Check sheet for the modelled part. Datum: model origin and axes. Units: mm. A direction names the side the tool comes from. Give positions to 0.01 mm unless a question says otherwise; leave off trailing zeros. Order: outer loops, then holes, each group sorted by start corner. A loop starts at its lowest first (then second) coordinate and runs counter-clockwise, first axis right, second up.
Item 1: Gauge pin test, flat ends, axial feed: P1, Ø0.6, axis at y = -0.5, z = 16.5, coming from the +X side; P2, Ø1.5, axis at y = 3, z = 7, coming from the +X side; P3, Ø1.6, axis at y = 0.5, z = 16.5, coming from the -X side. Record the tip position at first contact, or that the pin passes through.
Item 2: Sectioned sample at D-D on z = 9.25. Record the boundary of the cut face in (x, y), and give its area (3 significant figures).
Item 3: Material ranges on line 1 along Z through (x, y) = (3.5, 4.75); line 2 along X through (y, z) = (-0.5, 16.5); line 3 along Z through (x, y) = (-1.25, 1), recorded low to high.
Item 4: Sectioned sample at B-B on y = 0. Record the boundary of the cut face in (x, z), and give its area (3 significant figures).
Item 5: Release check for a two-part mould opening along X. For faces 6 (the cylindrical face through (-6, 0, 7)), 7 (the cylindrical face through (6, 0, 7)), 8 (the cylindrical face through (-0.54, -2.44, 15.49)) record: released by +X, released by -X, zero draft, split by the parting line, or undercut.
Item 6: Access from +Z, -Z, +X, -X, +Y, -Y to the whole of each face (thin tool, end or side, straight path). Record for faces 1 (the flat face through (-0.1, -2.2, 0)), 2 (the flat face through (-4.5, 0, 16)), 3 (the flat face through (3, 0, 15)), 4 (the flat face through (4.5, 0, 16)), 5 (the flat face through (4, 0, 16)).
Item 7: Sectioned sample at C-C on x = 0. Record the boundary of the cut face in (y, z), and give its area (3 significant figures).
Item 8: Sectioned sample at A-A on z = 15.5. Record the boundary of the cut face in (x, y), and give its area (3 significant figures).
from build123d import *

# Parameters (mm, degrees)
SKETCH_1_R          = 6
EXTRUDE_1_DEPTH     = 15
CUT_EXTRUDE_1_DEPTH = 15
SKETCH_7_R          = 2.5
EXTRUDE_2_DEPTH     = 1.2
FILLET_1_R          = 0.2
SKETCH_8_R          = 0.5
EXTRUDE_3_DEPTH     = 0.3
FILLET_2_R          = 0.05
EXTRUDE_4_DEPTH     = 2.4
CHAMFER_1_SIZE      = 0.5
CHAMFER_2_SIZE      = 0.5
CHAMFER_3_SIZE      = 0.5
SKETCH_10_R         = 2
EXTRUDE_5_DEPTH     = 0.1


with BuildPart() as part:
    # 草图1 → 凸台-拉伸1 (new body)
    with BuildSketch(Plane.XY):
        Circle(SKETCH_1_R)
    extrude(amount=EXTRUDE_1_DEPTH)

    # 草图6 → 切除-拉伸1 (cut)
    with BuildSketch(Plane(origin=(0, 0, 0), x_dir=(-1, 0, 0), z_dir=(0, 0, -1))):
        with BuildLine():
            Line((-3.31662479, 5), (3.31662479, 5))
            ThreePointArc((3.31662479, 5), (0, 6), (-3.31662479, 5))
        make_face()
        with BuildLine():
            Line((-3.31662479, -5), (3.31662479, -5))
            ThreePointArc((3.31662479, -5), (0, -6), (-3.31662479, -5))
        make_face()
    extrude(amount=-CUT_EXTRUDE_1_DEPTH, mode=Mode.SUBTRACT)

    # 草图7 → 凸台-拉伸2 (add)
    with BuildSketch(Plane.XY.offset(15)):
        Circle(SKETCH_7_R)
    extrude(amount=EXTRUDE_2_DEPTH)

    # 圆角1
    fillet_1_edges = [part.edges().sort_by_distance(p)[0] for p in [
        (-2.5, 0, 16.2),
    ]]
    fillet(fillet_1_edges, radius=FILLET_1_R)

    # 草图8 → 凸台-拉伸3 (add)
    with BuildSketch(Plane.XY.offset(16.2)):
        Circle(SKETCH_8_R)
    extrude(amount=EXTRUDE_3_DEPTH)

    # 圆角2
    fillet_2_edges = [part.edges().sort_by_distance(p)[0] for p in [
        (-0.5, 0, 16.5),
    ]]
    fillet(fillet_2_edges, radius=FILLET_2_R)

    # 草图9 → 凸台-拉伸4 (add)
    with BuildSketch(Plane.XY.offset(15)):
        Polygon((4, 0), (4, 1), (4.5, 1), (4.5, -1), (4, -1), align=None)
        Polygon((-4, -1), (-4, 0), (-4, 1), (-4.5, 1), (-4.5, -1), align=None)
    extrude(amount=EXTRUDE_4_DEPTH)

    # 倒角1
    chamfer_1_edges = [part.edges().sort_by_distance(p)[0] for p in [
        (-4.25, 1, 17.4),
    ]]
    chamfer(chamfer_1_edges, length=CHAMFER_1_SIZE)

    # 倒角2
    chamfer_2_edges = [part.edges().sort_by_distance(p)[0] for p in [
        (-4.25, -1, 17.4),
    ]]
    chamfer(chamfer_2_edges, length=CHAMFER_2_SIZE)

    # 倒角3
    chamfer_3_edges = [part.edges().sort_by_distance(p)[0] for p in [
        (4.25, -1, 17.4),
        (4.25, 1, 17.4),
    ]]
    chamfer(chamfer_3_edges, length=CHAMFER_3_SIZE)

    # 草图10 → 凸台-拉伸5 (add)
    with BuildSketch(Plane(origin=(0, 0, 0), x_dir=(-1, 0, 0), z_dir=(0, 0, -1))):
        Circle(SKETCH_10_R)
    extrude(amount=EXTRUDE_5_DEPTH)


solid = part.part
Report:
1. P1: stops at x = 4.5
1. P2: stops at x = 5.56
1. P3: stops at x = -4.5
2. outline: (-3.32, -5) - (3.32, -5) arc R6 ccw to (3.32, 5) - (-3.32, 5) arc R6 ccw to start
2. area: 104 mm2
3. line 1: z = 0 to 15
3. line 2: x = -4.5 to -4, 4 to 4.5
3. line 3: z = -0.1 to 16.2
4. outline: (-6, 0) - (-2, 0) - (-2, -0.1) - (2, -0.1) - (2, 0) - (6, 0) - (6, 15) - (4.5, 15) - (4.5, 17.4) - (4, 17.4) - (4, 15) - (2.5, 15) - (2.5, 16) arc R0.2 ccw to (2.3, 16.2) - (0.5, 16.2) - (0.5, 16.45) arc R0.05 ccw to (0.45, 16.5) - (-0.45, 16.5) arc R0.05 ccw to (-0.5, 16.45) - (-0.5, 16.2) - (-2.3, 16.2) arc R0.2 ccw to (-2.5, 16) - (-2.5, 15) - (-4, 15) - (-4, 17.4) - (-4.5, 17.4) - (-4.5, 15) - (-6, 15) - close
4. area: 189 mm2
5. face 6: released by -X
5. face 7: released by +X
5. face 8: undercut
6. face 1: -Z
6. face 2: +Z, -X, +Y, -Y
6. face 3: +Z
6. face 4: +Z, +X, +Y, -Y
6. face 5: +Z, +Y, -Y
7. outline: (-5, 0) - (-2, 0) - (-2, -0.1) - (2, -0.1) - (2, 0) - (5, 0) - (5, 15) - (2.5, 15) - (2.5, 16) arc R0.2 ccw to (2.3, 16.2) - (0.5, 16.2) - (0.5, 16.45) arc R0.05 ccw to (0.45, 16.5) - (-0.45, 16.5) arc R0.05 ccw to (-0.5, 16.45) - (-0.5, 16.2) - (-2.3, 16.2) arc R0.2 ccw to (-2.5, 16) - (-2.5, 15) - (-5, 15) - close
7. area: 157 mm2
8. outline: (-4.5, -1) - (-4, -1) - (-4, 1) - (-4.5, 1) - close; circle Ø5 at (0, 0); (4, -1) - (4.5, -1) - (4.5, 1) - (4, 1) - close
8. area: 21.6 mm2
